```python
from build123d import *

# Parameters (mm, degrees)
PAD_DEPTH          = 13
POCKET_DEPTH       = 3
POLARPATTERN_COUNT = 6
POCKET001_DEPTH    = 2


with BuildPart() as part:
    # Sketch → Pad (new body)
    with BuildSketch(Plane.XY):
        Polygon((0, 14.9), (8.6025190109, 14.9), (12.9037785164, 7.45), (12.0377531126, 6.95), (8.0251687417, 13.9), (0, 13.9), align=None)
    pad = extrude(amount=PAD_DEPTH)

    # Sketch001 → Pocket (cut)
    with BuildSketch(Plane.XY):
        Polygon((6.5, 11.2583302492), (11.7753229775, 14.3040393903), (6.5, 17.3497485314), align=None)
    pocket = extrude(amount=POCKET_DEPTH, mode=Mode.SUBTRACT)

    # PolarPattern: Pad, Pocket ×6 about axis
    polarpattern_axis = Axis((0, 0, 0), (0, 0, 1))
    for i in range(1, POLARPATTERN_COUNT):
        add(pad.rotate(polarpattern_axis, i * 360 / POLARPATTERN_COUNT))
        add(pocket.rotate(polarpattern_axis, i * 360 / POLARPATTERN_COUNT), mode=Mode.SUBTRACT)

    # Sketch002 (on Face50 of PolarPattern) → Pocket001 (cut)
    with BuildSketch(Plane.XZ.offset(14.9)):
        with BuildLine():
            ThreePointArc((1.7, 5), (0, 6.7), (-1.7, 5))
            Line((-1.7, 5), (-1.7, 0))
            Line((-1.7, 0), (1.7, 0))
            Line((1.7, 0), (1.7, 5))
        make_face()
    extrude(amount=-POCKET001_DEPTH, mode=Mode.SUBTRACT)


solid = part.part
```
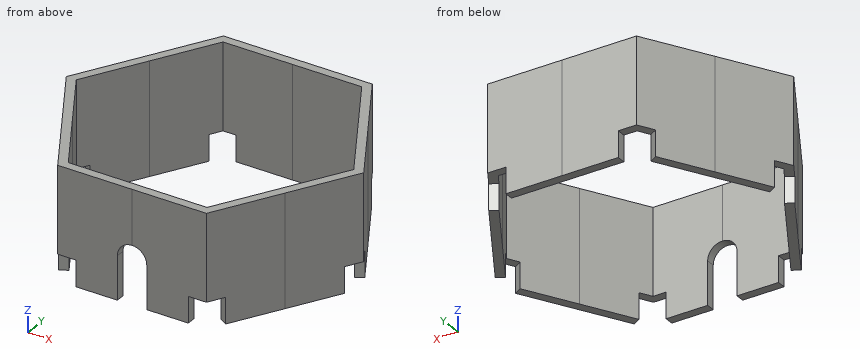
Here's how the part is built. I have some questions about the finished solid (model axes, mm). Round coordinates to 2 decimals unless told otherwise and drop trailing zeros. Write each loop counter-clockwise with the first axis right and the second up, starting at its lowest first coordinate (ties: lowest second). Pieces come first, ordered by that corner, then holes.
Q1. If we section it at A-A on x = -2.5: Write out the boundary of the cut face in (y, z), plus the area to 3 significant figures.
Q2. If we section it at B-B on z = 9.5: Write out the boundary of the cut face in (x, y), plus the area to 3 significant figures.
Q3. Please list where these lines run through material, in increasing order: probe 1 along Y at (x, z) = (-7.5, 10); probe 2 along Y at (x, z) = (8.5, 3.25); probe 3 along X at (y, z) = (5.5, 11.75).
Q4. Will these pins go through, and if not, where does the flat tip stop? P1, Ø0.7, axis at x = 7.5, y = -13.5, coming from the -Z side; P2, Ø0.5, axis at y = -14.5, z = 2, coming from the +X side; P3, Ø2.5, axis at x = -8.5, y = -14, coming from the -Z side; P4, Ø0.5, axis at y = -14.5, z = 1, coming from the -X side.
Q5. If we section it at C-C on y = -9.5: Write out the boundary of the cut face in (x, z).
Answer below:
1. outline: (-14.9, 0) - (-13.9, 0) - (-13.9, 13) - (-14.9, 13) - close; (13.9, 0) - (14.9, 0) - (14.9, 13) - (13.9, 13) - close
1. area: 26.0 mm2
2. outline: (-17.21, 0) - (-8.6, -14.9) - (8.6, -14.9) - (17.21, 0) - (8.6, 14.9) - (-8.6, 14.9) - close; hole (-16.05, 0) - (-8.03, -13.9) - (8.03, -13.9) - (16.05, 0) - (8.03, 13.9) - (-8.03, 13.9) - close
2. area: 99.8 mm2
3. probe 1: y = -14.9 to -13.9, 13.9 to 14.9
3. probe 2: y = -14.9 to -13.08, 13.08 to 14.9
3. probe 3: x = -14.03 to -12.87, 12.87 to 14.03
4. P1: passes through
4. P2: stops at x = 6.5
4. P3: stops at z = 3
4. P4: stops at x = -6.5
5. outline: (-11.72, 0) - (-10.57, 0) - (-10.57, 13) - (-11.72, 13) - close; (10.57, 0) - (11.72, 0) - (11.72, 13) - (10.57, 13) - close
